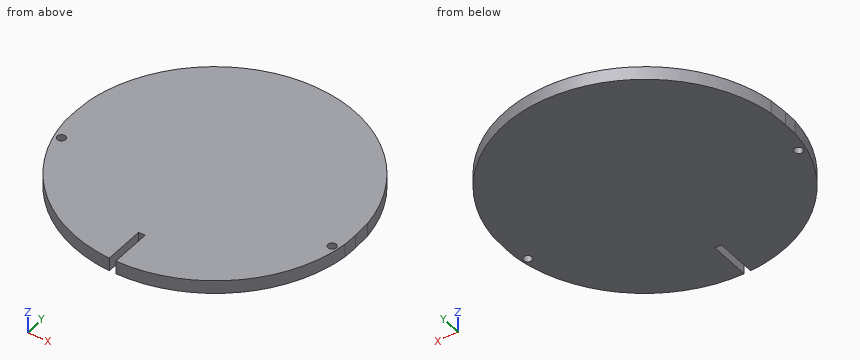
from build123d import *

# Parameters (mm, degrees)
BOSS_EXTRUDE1_DEPTH = 3.175
SKETCH2_R           = 1
CUT_EXTRUDE1_DEPTH  = 3.175
CUT_EXTRUDE2_DEPTH  = 3.175


with BuildPart() as part:
    # Sketch1 → Boss-Extrude1 (new body)
    with BuildSketch(Plane.XY.offset(377.209374622)):
        with BuildLine():
            Line((-33.799525455, -0.017072147), (-33.740147252, -3.418847174))
            add(Edge.make_bspline(
                [(-33.740147252, -3.418847174), (-33.521913435, -5.496739744), (-33.121758608, -7.52360336), (-32.245655467, -10.48651683), (-31.738647045, -11.948631126), (-31.127755378, -13.381606109), (-30.697366268, -14.330435347), (-30.470378572, -14.801900059), (-29.290211733, -17.119612441), (-27.644930506, -19.740333777), (-25.646898465, -22.113857284), (-24.588376817, -23.258919171), (-24.224726915, -23.634521718), (-23.482012785, -24.367327148), (-21.59014774, -26.150424449), (-18.705670827, -28.317861845), (-15.980786711, -29.823605713), (-14.107006772, -30.74768667), (-13.152701084, -31.164175695), (-10.256242476, -32.27934775), (-7.777960893, -32.988270972), (-5.214339656, -33.405899808), (-4.181967985, -33.549320099), (-3.661328308, -33.60925586), (-2.104532681, -33.751997759), (-1.069213869, -33.798542764), (2.029597644, -33.801687472), (4.085962141, -33.622116253), (7.155117004, -33.058726493), (8.178081257, -32.820670852), (10.177000978, -32.256577633), (11.158104767, -31.929888742), (14.04936497, -30.823232748), (15.907936031, -29.917809181), (18.13673294, -28.556406158), (18.576889104, -28.273087614), (19.438710135, -27.689460729), (20.706973253, -26.786573761), (21.903631517, -25.803366446), (23.438553372, -24.424422105), (24.544411843, -23.339363165), (25.578640539, -22.173955923), (26.251776296, -21.378677652), (26.580969723, -20.970778515), (28.17094662, -18.902925334), (29.269671397, -17.152899222), (30.678907287, -14.395868232), (31.108821176, -13.454846631), (31.884053374, -11.526054988), (32.230015293, -10.534907216), (33.119638114, -7.539302803), (33.521651228, -5.499562958), (33.740182048, -3.418847117)],
                knots=[0, 0, 0, 0, 0.0625, 0.0625, 0.09375, 0.109375, 0.109375, 0.125, 0.125, 0.1875, 0.21875, 0.21875, 0.234375, 0.234375, 0.25, 0.3125, 0.34375, 0.34375, 0.375, 0.375, 0.4375, 0.453125, 0.453125, 0.46875, 0.46875, 0.5, 0.5, 0.5625, 0.5625, 0.59375, 0.59375, 0.625, 0.625, 0.6875, 0.6875, 0.703125, 0.703125, 0.71875, 0.75, 0.75, 0.78125, 0.796875, 0.796875, 0.8125, 0.8125, 0.875, 0.875, 0.90625, 0.90625, 0.9375, 0.9375, 1, 1, 1, 1], degree=3))
            Line((33.740182048, -3.418847117), (33.799560251, -0.017072147))
            Line((33.799560251, -0.017072147), (33.560412457, 4.546139609))
            add(Edge.make_bspline(
                [(33.560412457, 4.546139609), (33.282065399, 6.567374379), (32.831372803, 8.534230691), (31.894626922, 11.402256897), (31.361087401, 12.815708643), (30.729491779, 14.19822173), (30.286610148, 15.113013144), (30.053701075, 15.567925007), (28.845742701, 17.805295292), (27.73617385, 19.487837269), (25.852855801, 21.84749908), (25.188593752, 22.606698061), (23.786460552, 24.069913543), (23.045059446, 24.776640829), (20.752328135, 26.778284029), (18.311067746, 28.558159122), (15.640647898, 29.995877244), (14.266739996, 30.656956524), (13.801141084, 30.868163008), (12.864758887, 31.267971853), (12.393699461, 31.456783193), (10.024605965, 32.347483289), (7.115279765, 33.1594713), (4.10232218, 33.57067126), (2.070213322, 33.754033964), (1.053662161, 33.799146951), (-1.978663229, 33.802802386), (-4.487220386, 33.587681269), (-6.97150073, 33.084409187), (-7.963243622, 32.859726611), (-8.459399615, 32.73533069), (-9.933669217, 32.329805435), (-10.897365307, 32.016750487), (-13.734609646, 30.957514861), (-15.554750033, 30.092235814), (-17.734673571, 28.798227251), (-18.165893543, 28.52880028), (-19.018645374, 27.968342063), (-19.439187613, 27.677889019), (-20.673952363, 26.783179445), (-21.465207676, 26.153069384), (-23.74871726, 24.167631397), (-25.151109466, 22.717611147), (-26.742507526, 20.734807748), (-27.053436756, 20.328702835), (-27.654958645, 19.504501759), (-28.525682186, 18.252011757), (-29.304349299, 16.952301265), (-30.745483656, 14.293275375), (-31.551336523, 12.44113352), (-32.506911863, 9.533039369), (-32.781055324, 8.547728647), (-33.237634192, 6.561909519), (-33.420905282, 5.558925362), (-33.560377664, 4.546139552)],
                knots=[0, 0, 0, 0, 0.0625, 0.0625, 0.09375, 0.109375, 0.109375, 0.125, 0.125, 0.1875, 0.1875, 0.21875, 0.21875, 0.25, 0.25, 0.3125, 0.34375, 0.34375, 0.359375, 0.359375, 0.375, 0.375, 0.4375, 0.46875, 0.46875, 0.5, 0.5, 0.5625, 0.578125, 0.578125, 0.59375, 0.59375, 0.625, 0.625, 0.6875, 0.6875, 0.703125, 0.703125, 0.71875, 0.71875, 0.75, 0.75, 0.8125, 0.8125, 0.828125, 0.828125, 0.84375, 0.875, 0.875, 0.9375, 0.9375, 0.96875, 0.96875, 1, 1, 1, 1], degree=3))
            Line((-33.560377664, 4.546139552), (-33.799525455, -0.017072147))
        make_face()
    extrude(amount=-BOSS_EXTRUDE1_DEPTH)

    # Sketch2 → Cut-Extrude1 (cut)
    with BuildSketch(Plane.XY.offset(377.209374622)):
        with Locations((32.009302375, -5.358989516)):
            Circle(SKETCH2_R)
        with Locations((-31.216064399, -8.164436653)):
            Circle(SKETCH2_R)
    extrude(amount=-CUT_EXTRUDE1_DEPTH, mode=Mode.SUBTRACT)

    # Sketch3 → Cut-Extrude2 (cut)
    with BuildSketch(Plane.XY.offset(377.209374622)):
        with BuildLine():
            Line((-0.018642697, -33.799604512), (-0.013127042, -23.799604512))
            Line((-0.013127042, -23.799604512), (-1.600627042, -23.799604512))
            Line((-1.600627042, -23.799604512), (-1.600627042, -33.762903096))
            add(Edge.make_bspline(
                [(-1.600627042, -33.762903096), (-1.078557444, -33.786966452), (-0.557114308, -33.799062449), (-0.030398621, -33.799596965), (-0.024520621, -33.79960146), (-0.018642697, -33.799604483)],
                knots=[0.484242822, 0.484242822, 0.484242822, 0.484242822, 0.5, 0.5, 0.500177833, 0.500177833, 0.500177833, 0.500177833], degree=3))
        make_face()
    extrude(amount=-CUT_EXTRUDE2_DEPTH, mode=Mode.SUBTRACT)


solid = part.part
The listing builds one solid part. Answer for the finished solid, in the listing's coordinates (mm). Give positions to 0.01 mm unless a question says otherwise; leave off trailing zeros. Use a Markdown table: item, result.
1. Section A-A on z = 376.55 is taken. Count the separate pieces of the cut face and the enclosed holes in it, plus the area to 3 significant figures.
Values follow:
| item | result |
|---|---|
| separate pieces | 1 |
| enclosed holes | 2 |
| area | 3,570 mm² |
2. Each of these flat-tipped pins is pushed along its axis until it touches: P1, Ø1, axis at y = 22, z = 374.5, coming from the +X side; P2, Ø1.5, axis at y = 9.5, z = 375, coming from the -X side. Where does it stop, or does it pass through?
Values follow:
| item | result |
|---|---|
| P1 | stops at x = 26.12 |
| P2 | stops at x = -32.71 |
3. Find the intervals of material crossed by probe 1 along X at (y, z) = (-30, 375.95); probe 2 along X at (y, z) = (-0.5, 374.95); probe 3 along X at (y, z) = (-27, 376.35), in increasing order. Write a range as from..to.
Values follow:
| item | result |
|---|---|
| probe 1 | x = -15.61..-1.6, -0.02..15.61 |
| probe 2 | x = -33.79..33.79 |
| probe 3 | x = -20.38..-1.6, -0.01..20.38 |
